from build123d import *

# Parameters (mm, degrees)
F1_DEPTH = 25.4
F2_W     = 5.954736
F2_H     = 12.7
F3_DEPTH = 8.255
F4_W     = 7.362218
F4_H     = 9.744114
F5_DEPTH = 12.7


with BuildPart() as f1:
    # F0 (on Front) → F1 (new body)
    with BuildSketch(Plane.XZ):
        Polygon((0, 22.952802), (0, 0), (37.135903, 0), (37.135903, 9.744114), (5.954736, 9.744114), (5.954736, 22.952802), align=None)
    extrude(amount=F1_DEPTH)

    # F2 (on face) → F3 (cut, symmetric)
    with BuildSketch(Plane.XY.offset(22.952802)):
        with Locations((2.977368, -12.7)):
            Rectangle(F2_W, F2_H)
    extrude(amount=F3_DEPTH, both=True, mode=Mode.SUBTRACT)

    # F4 (on face) → F5 (cut, symmetric)
    with BuildSketch(Plane.YZ.offset(37.135903)):
        with Locations((-12.450812, 4.872057)):
            Rectangle(F4_W, F4_H)
    extrude(amount=F5_DEPTH, both=True, mode=Mode.SUBTRACT)


solid = f1.part
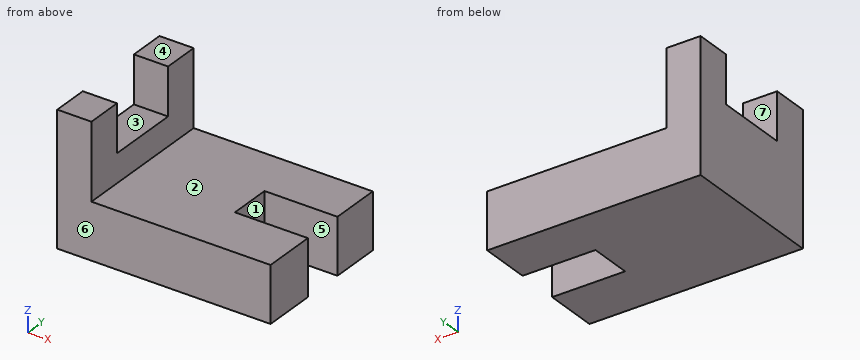
Read the model definition and answer for the solid it produces. Units are mm, in the model's axes. Face numbers are marked on the shaded views. A direction names the side the tool comes from. Coordinates: 2 decimals unless noted, no trailing zeros. Order: outer loops, then holes, each group sorted by start corner. A loop starts at its lowest first (then second) coordinate and runs counter-clockwise, first axis right, second up. Notation, with made-up numbers: M 7.5,50.5 L 54.5,50.5 A18 cw 54.5,85.5 Z; hole C 49.25,45.25 d2. An arc over 180 degrees is marked long. Put each result on its own line as item: value. Start each with the question number.
Item 1: Section D-D, the plane z = 8.25 is taken. Determine the outline of the cut face in (x, y).
Item 2: Section A-A, the plane x = 25 is taken. Determine the outline of the cut face in (y, z).
Item 3: Given pin 1 Ø3 at (x, y) = (2, -11) entering from +Z; pin 2 Ø12 at (y, z) = (-6.5, 18) entering from -X; pin 3 Ø4 at (x, y) = (18.5, -17.5) entering from +Z; pin 4 Ø2 at (y, z) = (-14, 4.5) entering from +X, each flat-ended and moving along its own axis, determine where each tip first touches the part or whether it passes through.
Item 4: For the marked faces 1, 2 and 3, determine the directions among +Z, -Z, +X, -X, +Y, -Y from which every point of the face is accessible in a straight line to the end or side of a thin tool.
Item 5: The mould has two halves that part along Y. Classify the marked faces 4, 5, 6 and 7: +Y half, -Y half, draft (parallel to the pull), parting line (faces both ways), or undercut.
Item 6: Section B-B, the plane z = 19.75 is taken. Determine the outline of the cut face in (x, y).
Item 7: Section C-C, the plane y = -15.25 is taken. Determine the outline of the cut face in (x, z), plus the area to 3 significant figures.
Item 8: Consider probe 1 along Y at (x, z) = (34.5, 8.75); probe 2 along Z at (x, y) = (33.5, -2.5); probe 3 along X at (y, z) = (-16, 11.75). Determine where each line is inside the solid, lowest interval first. Write a range as [from, to].
Computed:
1. outline: M 0,-25.4 L 37.14,-25.4 L 37.14,-16.13 L 24.44,-16.13 L 24.44,-8.77 L 37.14,-8.77 L 37.14,0 L 0,0 Z
2. outline: M -25.4,0 L -16.13,0 L -16.13,9.74 L -25.4,9.74 Z; M -8.77,0 L 0,0 L 0,9.74 L -8.77,9.74 Z
3. pin 1: stops at z = 14.7
3. pin 2: stops at x = 0
3. pin 3: stops at z = 9.74
3. pin 4: stops at x = 24.44
4. face 1: +Z, -Z, +X
4. face 2: +Z, +X, +Y, -Y
4. face 3: +Z, +X, -X
5. face 4: draft
5. face 5: undercut
5. face 6: -Y half
5. face 7: undercut
6. outline: M 0,-25.4 L 5.95,-25.4 L 5.95,-19.05 L 0,-19.05 Z; M 0,-6.35 L 5.95,-6.35 L 5.95,0 L 0,0 Z
7. outline: M 0,0 L 24.44,0 L 24.44,9.74 L 5.95,9.74 L 5.95,14.7 L 0,14.7 Z
7. area: 268 mm2
8. probe 1: y = [-25.4, -16.13], [-8.77, 0]
8. probe 2: z = [0, 9.74]
8. probe 3: x = [0, 5.95]
